Can you work these out from the model? Positions are in its coordinate system, mm. A direction names the side the tool comes from. Give positions to 0.01 mm unless a question says otherwise; leave off trailing zeros. Order: outer loops, then holes, each group sorted by start corner. A loop starts at its lowest first (then second) coordinate and runs counter-clockwise, first axis right, second up.
Item 1: I want a section at A-A, the plane z = 5.25. Write out the boundary of the cut face in (x, y), then the cut area to 3 significant figures.
Item 2: Which directions (+Z, -Z, +X, -X, +Y, -Y) give clear straight access to the entire face, cutting with the end or side of a thin tool? Please do faces 1 (the cylindrical face through (27.2, 24.99, 3.13)), 2 (the flat face through (41, -12.7, 3)).
Item 3: If we mould it in two halves opening along X, with no side actions, what happens to faces 3 (the flat face through (32, 4, 0)), 4 (the flat face through (25.4, -19, 3)), 5 (the flat face through (81.28, -13, 3))? For each: +X half, -X half, draft (parallel to the pull), parting line (faces both ways), or undercut.
Item 4: I want a section at C-C, the plane y = 42.5. Write out the boundary of the cut face in (x, z), then the cut area to 3 significant figures.
Item 5: I want a section at B-B, the plane x = 18. Write out the boundary of the cut face in (y, z), then the cut area to 3 significant figures.
Item 6: If I drill on line 1 along X through (y, z) = (-18, 2.25); line 2 along Y through (x, z) = (63, 5.75); line 3 along Y through (x, z) = (26.5, 1), over which ranges is the centre line in solid material (lowest first)?
Item 7: I'm going to push flat-ended pins straight in: pin 1 Ø3 at (x, z) = (55, 2.5) entering from +Y; pin 2 Ø3 at (y, z) = (35, 1.5) entering from +X; pin 3 Ø1.9 at (x, z) = (37, 4.5) entering from -Y. Where does each tip first touch, or does it pass through?
```python
from build123d import *

# Parameters (mm, degrees)
BOSS_EXTRUDE1_DEPTH = 6.35


with BuildPart() as part:
    # Sketch1 → Boss-Extrude1 (new body)
    with BuildSketch(Plane.XY):
        with BuildLine():
            ThreePointArc((0, 76.2), (27.810396475, 24.415089573), (81.28, 0))
            Line((81.28, 0), (0, 0))
            Line((0, 0), (0, 76.2))
        make_face()
        Polygon((0, -25.4), (0, 0), (81.28, 0), (81.28, -25.4), (55.88, -25.4), (55.88, -12.7), (25.4, -12.7), (25.4, -25.4), align=None)
    extrude(amount=BOSS_EXTRUDE1_DEPTH)


solid = part.part
```
Results list:
1. outline: (0, -25.4) - (25.4, -25.4) - (25.4, -12.7) - (55.88, -12.7) - (55.88, -25.4) - (81.28, -25.4) - (81.28, 0) arc R92.09 cw to (0, 76.2) - close
1. area: 3,350 mm2
2. face 1: +Z, -Z, +X, +Y
2. face 2: +Z, -Z, -Y
3. face 3: draft
3. face 4: undercut
3. face 5: +X half
4. outline: (0, 0) - (12.88, 0) - (12.88, 6.35) - (0, 6.35) - close
4. area: 81.8 mm2
5. outline: (-25.4, 0) - (35.19, 0) - (35.19, 6.35) - (-25.4, 6.35) - close
5. area: 385 mm2
6. line 1: x = 0 to 25.4, 55.88 to 81.28
6. line 2: y = -25.4 to 3.8
6. line 3: y = -12.7 to 25.67
7. pin 1: stops at y = 7.4
7. pin 2: stops at x = 19.34
7. pin 3: stops at y = -12.7
